Check sheet for the modelled part. Datum: model origin and axes. Units: mm. A direction names the side the tool comes from. Coordinates: 2 decimals unless noted, no trailing zeros. Loops run counter-clockwise (first coordinate to the right, second up) from the corner with the lowest first, then second, coordinate; pieces in that order, holes last. Notation, with made-up numbers: (-15.75, -8.75) -> (1.25, -8.75) arc R24 cw to (1.25, 26.25) -> close; hole circle Ø1 at (86, 36.5). An arc over 180 degrees is marked (long way). Use CSV: the item, a comma, the result in double quotes. Start each with the question number.
1. Sectioned sample at C-C, the plane x = 3. Record the cut outline in (y, z).
2. Sectioned sample at A-A, the plane z = 35.5. Record the cut outline in (x, y).
3. Set-up check for faces 1 (the face through (12.4, 4.6, 2)), 2 (the face through (5, 0, 40)): record each of +Z, -Z, +X, -X, +Y, -Y from which the full face is reachable in a straight line by a thin tool's end or side.
4. Gauge pin test, flat ends, axial feed: pin 1 (5 mm diameter, centred on x = -0.5, y = -2.5, fed in from -Z); pin 2 (8 mm diameter, centred on y = 12, z = 40.5, fed in from +X). Record the tip position at first contact, or that the pin passes through.
5. Release check for a two-part mould opening along X. For faces 3 (the face through (5, 5, 25)), 4 (the face through (12.4, 12.2, 31.3)), 5 (the face through (-5, 5, 31)) record: pulls with the +X half, pulls with the -X half, needs draft (parallel to the pull), parting line crosses it, or undercut.
6. Sectioned sample at D-D, the plane y = 2.5. Record the cut outline in (x, z).
7. Sectioned sample at B-B, the plane z = 16.5. Record the cut outline in (x, y), and give its area (3 significant figures).
8. Thickness scan on L1, parallel to X at y = 7, z = 38; L2, parallel to Y at x = 2, z = 36; L3, parallel to Z at x = 5.25, y = 7. Record the ranges inside material, lowest first.
```python
from build123d import *

# Parameters (mm, degrees)
SKETCH1_W           = 19.5
SKETCH1_H           = 19.2
SKETCH1_W_2         = 9.5
SKETCH1_H_2         = 9.2
BOSS_EXTRUDE1_DEPTH = 55
SKETCH1_2_W         = 9.5
SKETCH1_2_H         = 9.2
BOSS_EXTRUDE2_DEPTH = 25
FILLET2_R           = 7


with BuildPart() as part:
    # Sketch1 → Boss-Extrude1 (new body)
    with BuildSketch(Plane.XY):
        with Locations((4.75, 4.6)):
            Rectangle(SKETCH1_W, SKETCH1_H)
        with Locations((4.75, 4.6)):
            Rectangle(SKETCH1_W_2, SKETCH1_H_2, mode=Mode.SUBTRACT)
    extrude(amount=BOSS_EXTRUDE1_DEPTH)

    # Sketch1<2> → Boss-Extrude2 (add)
    with BuildSketch(Plane.XY):
        with Locations((4.75, 4.6)):
            Rectangle(SKETCH1_2_W, SKETCH1_2_H)
    extrude(amount=BOSS_EXTRUDE2_DEPTH)

    # Fillet2
    fillet2_edges = [part.edges().sort_by_distance(p)[0] for p in [
        (4.75, 14.2, 0),
        (14.5, 4.6, 0),
        (4.75, -5, 0),
        (-5, 4.6, 0),
        (-5, 14.2, 27.5),
        (14.5, 14.2, 27.5),
        (14.5, -5, 27.5),
        (-5, -5, 27.5),
    ]]
    fillet(fillet2_edges, radius=FILLET2_R)


solid = part.part
```
Completed:
1,outline,"(-5, 7) arc R7 ccw to (2, 0) -> (7.2, 0) arc R7 ccw to (14.2, 7) -> (14.2, 55) -> (9.2, 55) -> (9.2, 25) -> (0, 25) -> (0, 55) -> (-5, 55) -> close"
2,outline,"(-5, 2) arc R7 ccw to (2, -5) -> (7.5, -5) arc R7 ccw to (14.5, 2) -> (14.5, 7.2) arc R7 ccw to (7.5, 14.2) -> (2, 14.2) arc R7 ccw to (-5, 7.2) -> close; hole (0, 0) -> (9.5, 0) -> (9.5, 9.2) -> (0, 9.2) -> close"
3,face 1,"-Z, +X, +Y, -Y"
3,face 2,"+Z"
4,pin 1,"z = 0.52"
4,pin 2,"x = 14.45"
5,face 3,"undercut"
5,face 4,"pulls with the +X half"
5,face 5,"pulls with the -X half"
6,outline,"(-5, 7) arc R7 ccw to (2, 0) -> (7.5, 0) arc R7 ccw to (14.5, 7) -> (14.5, 55) -> (9.5, 55) -> (9.5, 25) -> (0, 25) -> (0, 55) -> (-5, 55) -> close"
7,outline,"(-5, 2) arc R7 ccw to (2, -5) -> (7.5, -5) arc R7 ccw to (14.5, 2) -> (14.5, 7.2) arc R7 ccw to (7.5, 14.2) -> (2, 14.2) arc R7 ccw to (-5, 7.2) -> close"
7,area,"332 mm²"
8,L1,"-5 to 0, 9.5 to 14.5"
8,L2,"-5 to 0, 9.2 to 14.2"
8,L3,"0 to 25"
